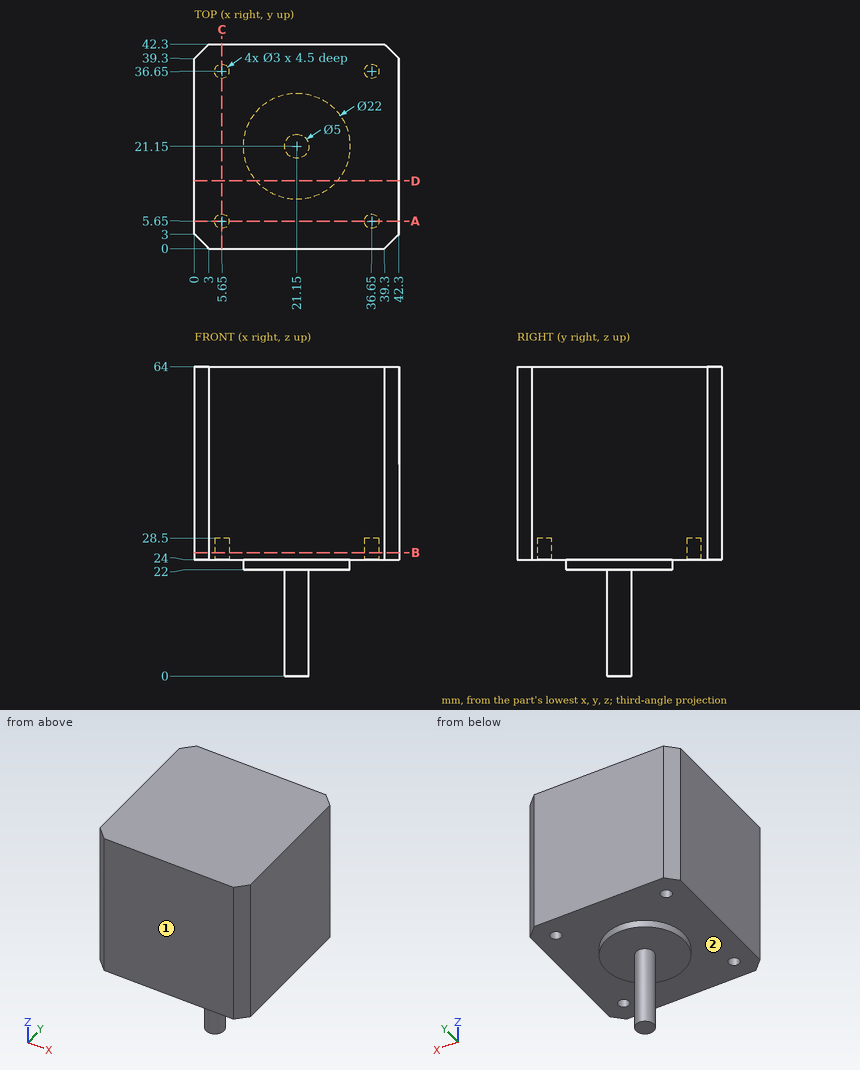
Could you check a few things on this drawing? It's one solid part, dimensions in mm from its lowest x, y, z. A direction names the side the tool comes from. Coordinates: 2 decimals unless noted, no trailing zeros. Write each loop counter-clockwise with the first axis right and the second up, starting at its lowest first coordinate (ties: lowest second). Pieces come first, ordered by that corner, then holes. Notation, with made-up numbers: (36, -37) - (56, -37) arc R15 ccw to (56, -18) - close; hole circle Ø4 at (24.25, 37.5). An arc over 180 degrees is marked (long way). Write item = value, one per line.
1) Suppose I cut it at A-A on y = 5.65. Please give me the cut outline in (x, z).
Result set:
outline = (0, 24) - (4.15, 24) - (4.15, 28.5) - (7.15, 28.5) - (7.15, 24) - (35.15, 24) - (35.15, 28.5) - (38.15, 28.5) - (38.15, 24) - (42.3, 24) - (42.3, 64) - (0, 64) - close
2) Will these pins go through, and if not, where does the flat tip stop? pin 1 Ø2.5 at (x, y) = (37, 5) entering from -Z; pin 2 Ø0.9 at (x, y) = (6, 37) entering from -Z; pin 3 Ø1.5 at (y, z) = (21, 22) entering from -X; pin 4 Ø11 at (x, y) = (26.5, 19.5) entering from -Z.
Result set:
pin_1 = 24
pin_2 = 28.5
pin_3 = 10.15
pin_4 = 0
3) Please list where these lines run through material, in increasing order: line 1 (X direction, y = 36.65, z = 27.05); line 2 (Y direction, x = 5, z = 26); line 3 (Z direction, x = 13, y = 18). Write a range as [from, to].
Result set:
line_1 = [0, 4.15], [7.15, 35.15], [38.15, 42.3]
line_2 = [0, 4.3], [7, 35.3], [38, 42.3]
line_3 = [22, 64]
4) Suppose I cut it at D-D on y = 14. Please give me the cut outline in (x, z).
Result set:
outline = (0, 24) - (12.79, 24) - (12.79, 22) - (29.51, 22) - (29.51, 24) - (42.3, 24) - (42.3, 64) - (0, 64) - close
5) For the marked faces 1 and 2, which set-ups out of +Z, -Z, +X, -X, +Y, -Y let a thin tool reach every point of the face, with its end or its side?
Result set:
face_1 = +Z, -Z, +X, -X, -Y
face_2 = -Z
6) Suppose I cut it at B-B on z = 25.5. Please give me the cut outline in (x, y), plus the area to 3 significant figures.
Result set:
outline = (0, 3) - (3, 0) - (39.3, 0) - (42.3, 3) - (42.3, 39.3) - (39.3, 42.3) - (3, 42.3) - (0, 39.3) - close; hole circle Ø3 at (5.65, 5.65); hole circle Ø3 at (5.65, 36.65); hole circle Ø3 at (36.65, 5.65); hole circle Ø3 at (36.65, 36.65)
area = 1,740 mm2
